```python
from build123d import *

# Parameters (mm, degrees)
SKETCH_1_W          = 245
SKETCH_1_H          = 55
SKETCH_1_R          = 16.5
SKETCH_1_R_2        = 2
SKETCH_1_R_3        = 3.5
SKETCH_1_R_4        = 10
EXTRUDE_4_DEPTH     = 10
SKETCH_2_R          = 5.5
CUT_EXTRUDE_1_DEPTH = 5.5
FILLET_1_R          = 1


with BuildPart() as part:
    # 草图1 → 凸台-拉伸4 (new body)
    with BuildSketch(Plane(origin=(0, 0, 0), x_dir=(1, 0, 0), z_dir=(0, 1, 0))):
        with Locations((122.617986059, 27.264027881)):
            Rectangle(SKETCH_1_W, SKETCH_1_H)
        with Locations(Location((32.5, 27.5, 0), (0, 0, 270))):
            Circle(SKETCH_1_R, mode=Mode.SUBTRACT)
        with Locations(Location((11, 27.5, 0), (0, 0, 270))):
            Circle(SKETCH_1_R_2, mode=Mode.SUBTRACT)
        with Locations(Location((54, 27.5, 0), (0, 0, 270))):
            Circle(SKETCH_1_R_2, mode=Mode.SUBTRACT)
        with Locations(Location((32.5, 6, 0), (0, 0, 270))):
            Circle(SKETCH_1_R_2, mode=Mode.SUBTRACT)
        with Locations(Location((72.5, 10, 0), (0, 0, 270))):
            Circle(SKETCH_1_R_3, mode=Mode.SUBTRACT)
        with Locations(Location((72.5, 45, 0), (0, 0, 270))):
            Circle(SKETCH_1_R_3, mode=Mode.SUBTRACT)
        with Locations(Location((32.5, 49, 0), (0, 0, 270))):
            Circle(SKETCH_1_R_2, mode=Mode.SUBTRACT)
        with Locations(Location((212.5, 6, 0), (0, 0, 270))):
            Circle(SKETCH_1_R_2, mode=Mode.SUBTRACT)
        with Locations(Location((172.5, 10, 0), (0, 0, 270))):
            Circle(SKETCH_1_R_3, mode=Mode.SUBTRACT)
        with Locations(Location((234, 27.5, 0), (0, 0, 270))):
            Circle(SKETCH_1_R_2, mode=Mode.SUBTRACT)
        with Locations(Location((191, 27.5, 0), (0, 0, 270))):
            Circle(SKETCH_1_R_2, mode=Mode.SUBTRACT)
        with Locations(Location((172.5, 45, 0), (0, 0, 270))):
            Circle(SKETCH_1_R_3, mode=Mode.SUBTRACT)
        with Locations(Location((212.5, 49, 0), (0, 0, 270))):
            Circle(SKETCH_1_R_2, mode=Mode.SUBTRACT)
        with Locations(Location((212.5, 27.5, 0), (0, 0, 270))):
            Circle(SKETCH_1_R, mode=Mode.SUBTRACT)
        with Locations(Location((122.5, 27.5, 0), (0, 0, 270))):
            Circle(SKETCH_1_R_4, mode=Mode.SUBTRACT)
    extrude(amount=EXTRUDE_4_DEPTH)

    # 草图2 → 切除-拉伸1 (cut)
    with BuildSketch(Plane(origin=(0, 10, 0), x_dir=(1, 0, 0), z_dir=(0, 1, 0))):
        with Locations(Location((72.5, 45, 0), (0, 0, 270))):
            Circle(SKETCH_2_R)
        with Locations(Location((72.5, 10, 0), (0, 0, 270))):
            Circle(SKETCH_2_R)
        with Locations(Location((172.5, 45, 0), (0, 0, 270))):
            Circle(SKETCH_2_R)
        with Locations(Location((172.5, 10, 0), (0, 0, 270))):
            Circle(SKETCH_2_R)
    extrude(amount=-CUT_EXTRUDE_1_DEPTH, mode=Mode.SUBTRACT)

    # 圆角1
    fillet_1_edges = [part.edges().sort_by_distance(p)[0] for p in [
        (0.117986059, 5, -54.764027881),
        (0.117986059, 5, 0.235972119),
        (245.117986059, 5, 0.235972119),
        (245.117986059, 5, -54.764027881),
    ]]
    fillet(fillet_1_edges, radius=FILLET_1_R)


solid = part.part
```
Check sheet for the modelled part. Datum: model origin and axes. Units: mm. A direction names the side the tool comes from. Round coordinates to 2 decimals unless told otherwise and drop trailing zeros. Order: outer loops, then holes, each group sorted by start corner. A loop starts at its lowest first (then second) coordinate and runs counter-clockwise, first axis right, second up. Notation, with made-up numbers: (-3.5, 52.25) -> (17.5, 52.25) arc R35 cw to (17.5, 91.25) -> close; hole circle Ø4 at (13, -31.5). An arc over 180 degrees is marked (long way). One line per item, written item: value. Start each with the question number.
Q1. Cross-section at B-B (x = 116). Record the boundary of the cut face in (y, z).
Q2. Gauge pin test, flat ends, axial feed: pin 1 Ø3.5 at (x, z) = (191, -27.5) entering from +Y; pin 2 Ø12.5 at (x, z) = (172.5, -10) entering from -Y. Record the tip position at first contact, or that the pin passes through.
Q3. Mould release check, pull along X, two halves, no side actions. Record for faces 3 (the face through (121, 10, -40)), 4 (the face through (73, 4.5, -6)), 5 (the face through (0.118, 5, -27)), 6 (the face through (210.726, 4.93, -48.077)): pulls with the +X half, pulls with the -X half, needs draft (parallel to the pull), parting line crosses it, or undercut.
Q4. Thickness scan on line 1 (X direction, y = 1.7, z = -10); line 2 (Z direction, x = 72.5, y = 1.5); line 3 (X direction, y = 8.1, z = -45). Record the ranges inside material, lowest first.
Q5. Cross-section at A-A (y = 8.25). Give the number of separate pieces and of enclosed holes in the cut face, and give its area (3 significant figures).
Q6. Set-up check for faces 1 (the face through (121, 0, -40)), 2 (the face through (167.13, 7.29, -11.19)): record each of +Z, -Z, +X, -X, +Y, -Y from which the full face is reachable in a straight line by a thin tool's end or side.
Q7. Cross-section at C-C (x = 46.5). Record the boundary of the cut face in (y, z), and give its area (3 significant figures).
Completed:
1. outline: (0, -54.76) -> (10, -54.76) -> (10, -35.1) -> (0, -35.1) -> close; (0, -19.9) -> (10, -19.9) -> (10, 0.24) -> (0, 0.24) -> close
2. pin 1: passes through
2. pin 2: stops at y = 0
3. face 3: needs draft
3. face 4: undercut
3. face 5: pulls with the -X half
3. face 6: undercut
4. line 1: x = 0.12 to 69, 76 to 169, 176 to 245.12
4. line 2: z = -54.76 to -48.5, -41.5 to -13.5, -6.5 to 0.24
4. line 3: x = 0.12 to 67, 78 to 167, 178 to 245.12
5. separate pieces: 1
5. enclosed holes: 15
5. area: 11,000 mm²
6. face 1: +Z, -Z, +X, -X, -Y
6. face 2: +Y
7. outline: (0, -54.76) -> (10, -54.76) -> (10, -36.23) -> (0, -36.23) -> close; (0, -18.77) -> (10, -18.77) -> (10, 0.24) -> (0, 0.24) -> close
7. area: 375 mm²
